Geometry check sheet. Reference: the model listing, model coordinates, mm. A direction names the side the tool comes from. Coordinates: 2 decimals unless noted, no trailing zeros. Write each loop counter-clockwise with the first axis right and the second up, starting at its lowest first coordinate (ties: lowest second). Pieces come first, ordered by that corner, then holes. Notation, with made-up numbers: M 86,83 L 97,83 A11 cw 97,96 Z; hole C -3,4.25 d4. An arc over 180 degrees is marked long. Write each question's results on one line, items separated by ' | '.
Autodesk Inventor part; units mm, degrees
ref_plane "YZ Plane" through (0, 0, 0) normal (1, 0, 0) x (0, 1, 0)
ref_plane "XZ Plane" through (0, 0, 0) normal (0, 1, 0) x (-1, 0, 0)
ref_plane "XY Plane" through (0, 0, 0) normal (0, 0, 1) x (1, 0, 0)
sketch "Sketch4" plane through (0, 0, 0) normal (0, 0, 1) x (1, 0, 0)
  line L0 (-10.5, 0) -> (10.5, 0)
  line L1 (0, -3.3) -> (0, 19.8)
  line L2 (-7.5, 0) -> (7.5, 0)
  line L3 (7.5, 0) -> (7.5, 16.5)
  line L4 (7.5, 16.5) -> (-7.5, 16.5)
  line L5 (-7.5, 16.5) -> (-7.5, 0)
  circle A0 centre (0, 10) radius 2.5
  point P0 (0, 0)
  dimension "d0" = 7.5
  dimension "d1" = 7.5
  dimension "d2" = 16.5
  dimension "d3" = 5
  dimension "d4" = 6.5
extrude "Extrusion1" add sketch "Sketch4" against normal blind 15.9 contours L5 L4 L1 A0 L0 | L1 A0 L4 L3 L0
fillet "Fillet1" radius 7.5 2 edges at (7.5, 16.5, -7.95) (-7.5, 16.5, -7.95)
sketch "Sketch5" plane through (-7.5, 0, 0) normal (0, -1, 0) x (1, 0, 0)
  line L0 (0, 0) -> (0, -15.9)
  line L1 (15, 0) -> (15, -15.9)
  line L2 (0, 0) -> (15, 0)
  line L3 (15, 0) -> (15, -15.9)
  line L4 (15, -15.9) -> (0, -15.9)
  line L5 (0, -15.9) -> (0, 0)
  point P0 (7.5, 0)
extrude "Extrusion2" add sketch "Sketch5" along normal blind 5
sketch "Sketch6" plane through (7.5, 9, 0) normal (1, 0, 0) x (0, 0, -1)
  point P0 (0, -9)
sketch "Sketch7" plane through (7.5, 9, 0) normal (1, 0, 0) x (0, 0, -1)
  line L0 (0, 0) -> (0, 7.5)
  line L1 (0, 7.5) -> (3.3, 7.5)
  line L2 (3.3, 7.5) -> (3.3, -7.5)
  line L3 (3.3, -7.5) -> (0, -7.5)
  line L4 (0, -7.5) -> (0, 7.5)
  line L5 (0, 7.5) -> (15.9, 7.5)
  line L6 (6.3, 7.5) -> (9.6, 7.5)
  line L7 (9.6, 7.5) -> (9.6, -7.5)
  line L8 (9.6, -7.5) -> (6.3, -7.5)
  line L9 (6.3, -7.5) -> (6.3, 7.5)
  line L10 (12.6, 7.5) -> (15.9, 7.5)
  line L11 (15.9, 7.5) -> (15.9, -7.5)
  line L12 (15.9, -7.5) -> (12.6, -7.5)
  line L13 (12.6, -7.5) -> (12.6, 7.5)
  line L14 (3.3, -7.5) -> (6.3, -7.5)
  line L15 (9.6, -7.5) -> (12.6, -7.5)
  line L16 (3.3, 7.5) -> (6.3, 7.5)
  line L17 (9.6, 7.5) -> (12.6, 7.5)
  point P0 (0, -9)
  dimension "d10" = 3.3
  dimension "d11" = 15
  dimension "d12" = 3
  dimension "d13" = 3.3
  dimension "d14" = 3
  dimension "d15" = 3.3
sketch "Sketch8" plane through (7.5, 9, 0) normal (1, 0, 0) x (0, 0, -1)
  line L0 (0, 7.5) -> (15.9, 7.5)
  line L1 (3.3, 7.5) -> (6.2995, 7.5)
  line L2 (6.2995, 7.5) -> (6.2995, -7.4999)
  line L3 (6.2995, -7.4999) -> (3.3, -7.4999)
  line L4 (3.3, -7.4999) -> (3.3, 7.5)
  line L5 (9.5994, 7.5) -> (12.5997, 7.5)
  line L6 (12.5997, 7.5) -> (12.5997, -7.4999)
  line L7 (12.5997, -7.4999) -> (9.5994, -7.4999)
  line L8 (9.5994, -7.4999) -> (9.5994, 7.5)
  point P0 (0, -9)
extrude "Extrusion3" cut sketch "Sketch7" against normal through all contours L5 L13 L15 L7
extrude "Extrusion4" cut sketch "Sketch8" against normal through all contours L0 L2 L3 L4
properties part number "gopro_base"
Q1. Scan lines: probe 1 along Z at (x, y) = (-1.5, 15.75); probe 2 along Y at (x, z) = (0, -2.1); probe 3 along Y at (x, z) = (-2.75, -10). Record each from-to range of solid material in increasing order.
Geometry check:
probe 1: z = -15.9 to -12.6, -9.6 to -6.3, -3.3 to 0 | probe 2: y = -5 to 7.5, 12.5 to 16.5 | probe 3: y = -5 to 1.5
Q2. Sectioned sample at B-B on x = -0.25. Record the cut outline in (y, z).
Geometry check:
outline: M -5,-15.9 L 7.51,-15.9 L 7.51,-12.6 L 1.5,-12.6 L 1.5,-9.6 L 7.51,-9.6 L 7.51,-6.3 L 1.5,-6.3 L 1.5,-3.3 L 7.51,-3.3 L 7.51,0 L -5,0 Z; M 12.49,-15.9 L 16.5,-15.9 L 16.5,-12.6 L 12.49,-12.6 Z; M 12.49,-9.6 L 16.5,-9.6 L 16.5,-6.3 L 12.49,-6.3 Z; M 12.49,-3.3 L 16.5,-3.3 L 16.5,0 L 12.49,0 Z
Q3. Sectioned sample at D-D on y = 11.25. Record the cut outline in (x, z).
Geometry check:
outline: M -7.15,-15.9 L -2.17,-15.9 L -2.17,-12.6 L -7.15,-12.6 Z; M -7.15,-9.6 L -2.17,-9.6 L -2.17,-6.3 L -7.15,-6.3 Z; M -7.15,-3.3 L -2.17,-3.3 L -2.17,0 L -7.15,0 Z; M 2.17,-15.9 L 7.15,-15.9 L 7.15,-12.6 L 2.17,-12.6 Z; M 2.17,-9.6 L 7.15,-9.6 L 7.15,-6.3 L 2.17,-6.3 Z; M 2.17,-3.3 L 7.15,-3.3 L 7.15,0 L 2.17,0 Z
Q4. Mould release check, pull along Z, two halves, no side actions. Record for faces 3 (the flat face through (0, 1.5, -5)), 4 (the cylindrical face through (5.245, 14.361, -1.673)), 5 (the flat face through (0, 6, 0)): pulls with the +Z half, pulls with the -Z half, needs draft (parallel to the pull), parting line crosses it, or undercut.
Geometry check:
face 3: undercut | face 4: needs draft | face 5: pulls with the +Z half
Q5. Sectioned sample at A-A on y = 5.5. Record the cut outline in (x, z).
Geometry check:
outline: M -7.5,-15.9 L 7.5,-15.9 L 7.5,-12.6 L -7.5,-12.6 Z; M -7.5,-9.6 L 7.5,-9.6 L 7.5,-6.3 L -7.5,-6.3 Z; M -7.5,-3.3 L 7.5,-3.3 L 7.5,0 L -7.5,0 Z
Q6. Access from +Z, -Z, +X, -X, +Y, -Y to the whole of each face (thin tool, end or side, straight path). Record for faces 1 (the flat face through (0, -5, -8)), 2 (the flat face through (0, 7, -3.3)).
Geometry check:
face 1: +Z, -Z, +X, -X, -Y | face 2: +X, -X, +Y
Q7. Depth check by flat-ended pin: P1, Ø5, axis at y = 12, z = -8, coming from the +X side; P2, Ø2.5, axis at x = -1, z = -4, coming from the +Y side; P3, Ø1.5, axis at x = 1, z = -11, coming from the +Y side. Enter the tip coordinate at first touch or a pass-through.
Geometry check:
P1: stops at x = 7.48 | P2: stops at y = 16.5 | P3: stops at y = 1.5
